from build123d import *

# Parameters (mm, degrees)
F0_W     = 25.4
F0_H     = 25.4
F1_DEPTH = 3.175
F1_TAPER = 25
F3_W     = 5.08
F3_H     = 12.7
F6_DEPTH = 6.35
F7_R     = 5.08


with BuildPart() as f1:
    # F0 (on Top) → F1 (new body)
    with BuildSketch(Plane.XY):
        Rectangle(F0_W, F0_H)
    extrude(amount=F1_DEPTH, taper=F1_TAPER)

    # F4: sweep along a path in F2
    with BuildLine(Plane.XZ) as f4_path:
        ThreePointArc((-10.16, 0), (0, -23.5582897328), (10.16, 0))
    # F3 (on face) → F4 (sweep)
    with BuildSketch(Plane(origin=(0, 0, 0), x_dir=(1, 0, 0), z_dir=(0, 0, -1))):
        with Locations((10.16, 0)):
            Rectangle(F3_W, F3_H)
    sweep(path=f4_path.line)

    # F5 (on Front) → F6 (join, symmetric)
    with BuildSketch(Plane.XZ):
        with BuildLine():
            Line((-7.62, 0), (-10.16, 0))
            Line((-10.16, 0), (-10.0130578512, -2.535746045))
            ThreePointArc((-10.0130578512, -2.535746045), (-8.9072265211, -1.1822790439), (-7.62, 0))
        make_face()
    extrude(amount=F6_DEPTH, both=True)

    # F7
    f7_edges = [f1.edges().sort_by_distance(p)[0] for p in [
        (-11.959737, 11.959737, 1.5875),
        (11.959737, 11.959737, 1.5875),
        (11.959737, -11.959737, 1.5875),
        (-11.959737, -11.959737, 1.5875),
    ]]
    fillet(f7_edges, radius=F7_R)


solid = f1.part
CAD build for the part. Positions are in the model's coordinates, mm. A direction names the side the tool comes from. Round coordinates to 2 decimals unless told otherwise and drop trailing zeros. Loops run counter-clockwise (first coordinate to the right, second up) from the corner with the lowest first, then second, coordinate; pieces in that order, holes last.
(1) Wall check: line 1 along Y through (x, z) = (-13.5, -8.25); line 2 along X through (y, z) = (0, -17); line 3 along X through (y, z) = (3.25, -16.5). Give the ranges that are in metal, low to high.
(2) Two-plate mould, pull along Z, no slides. Class faces 3 (the cylindrical face through (-10.52, -10.59, 1.81)), 4 (the flat face through (0, 0, 0)), 5 (the flat face through (0, -6.35, -22)), 6 (the cylindrical face through (-0.494, -0.089, -25.494)): +Z half, -Z half, draft (parallel to the pull), parting line (faces both ways), or undercut.
(3) Drop flat-ended pins along their axis: pin 1 (1.5 mm diameter, centred on y = -6, z = -17, fed in from -X); pin 2 (13 mm diameter, centred on x = 6, z = -11.5, fed in from +Y); pin 3 (3 mm diameter, centred on y = -5, z = -18, fed in from +X). Give the stop position or say it passes through.
(4) Cut at D-D (z = -24). Give the cut face in (x, y).
(5) Cut at C-C (z = -20.5). Give the cut face in (x, y).
(6) Which spindle directions (+Z, -Z, +X, -X, +Y, -Y) get a long thin tool onto all of the face, cutting with end or side? Do faces 1 (the flat face through (0.11, -11.97, 1.57)), 2 (the flat face through (0, 6.35, -22)). Say none if no direction does.
(7) Cut at B-B (y = 3). Give the cut face in (x, z) (3 decimals).
(8) Cut at A-A (x = 0). Give the cut face in (y, z) (3 decimals), plus the area to 3 significant figures.
Findings below:
1. line 1: y = -6.35 to 6.35
1. line 2: x = -14.08 to -9.75, 9.75 to 14.08
1. line 3: x = -14.33 to -10.11, 10.11 to 14.33
2. face 3: +Z half
2. face 4: undercut
2. face 5: draft
2. face 6: parting line
3. pin 1: stops at x = -14.45
3. pin 2: stops at y = 6.35
3. pin 3: stops at x = 14.33
4. outline: (-6.75, -6.35) - (6.75, -6.35) - (6.75, 6.35) - (-6.75, 6.35) - close
5. outline: (-11.58, -6.35) - (-5.56, -6.35) - (-5.56, 6.35) - (-11.58, 6.35) - close; (5.56, -6.35) - (11.58, -6.35) - (11.58, 6.35) - (5.56, 6.35) - close
6. face 1: +Z, +X, -X, -Y
6. face 2: -Z, +X, -X, +Y
7. outline: (-12.7, 0) arc R15.913 ccw (long way) to (12.7, 0) - (11.219, 3.175) - (-11.219, 3.175) - close; hole (-7.62, 0) arc R12.247 ccw (long way) to (7.62, 0) - close
8. outline: (-12.7, 0) - (12.7, 0) - (11.219, 3.175) - (-11.219, 3.175) - close; (-6.35, -25.501) - (6.35, -25.501) - (6.35, -21.836) - (-6.35, -21.836) - close
8. area: 122 mm2
